The model under review builds one solid part; all positions refer to its coordinate system, in mm. Face numbers are marked on the shaded views. Round coordinates to 2 decimals unless told otherwise and drop trailing zeros. Order: outer loops, then holes, each group sorted by start corner. A loop starts at its lowest first (then second) coordinate and runs counter-clockwise, first axis right, second up. Notation, with made-up numbers: M 2.25,42.25 L 61.25,42.25 A23 cw 61.25,55.25 Z; hole C -25,-8.5 d7. An arc over 180 degrees is marked long. One line per item, written item: value. Start each with the question number.
from build123d import *

# Parameters (mm, degrees)
F0_R     = 1.6
F1_DEPTH = 3.175


with BuildPart() as f1:
    # F0 (on Top) → F1 (new body)
    with BuildSketch(Plane.XY):
        with BuildLine():
            Line((38.1, 6.35), (0, 6.35))
            ThreePointArc((0, 6.35), (-4.490128, 4.490128), (-6.35, 0))
            ThreePointArc((-6.35, 0), (-4.490128, -4.490128), (0, -6.35))
            Line((0, -6.35), (38.1, -6.35))
            ThreePointArc((38.1, -6.35), (42.590128, -4.490128), (44.45, 0))
            ThreePointArc((44.45, 0), (42.590128, 4.490128), (38.1, 6.35))
        make_face()
        with Locations((8.1, -3.175)):
            Circle(F0_R, mode=Mode.SUBTRACT)
        with Locations((18.1, -3.175)):
            Circle(F0_R, mode=Mode.SUBTRACT)
        with Locations((28.1, -3.175)):
            Circle(F0_R, mode=Mode.SUBTRACT)
        with Locations((38.1, -3.175)):
            Circle(F0_R, mode=Mode.SUBTRACT)
        Polygon((-2.313127, 1.150841), (-2.481189, 1.651718), (-1.954254, 1.689937), (-1.992473, 2.216873), (-1.472587, 2.122848), (-1.378562, 2.642733), (-0.898392, 2.422372), (-0.678031, 2.902541), (-0.267748, 2.56969), (0.065104, 2.979972), (0.37972, 2.555544), (0.804147, 2.87016), (1.003328, 2.380825), (1.492663, 2.580005), (1.563894, 2.056509), (2.08739, 2.12774), (2.026194, 1.602976), (2.550958, 1.54178), (2.361181, 1.048721), (2.85424, 0.858945), (2.547807, 0.428572), (2.97818, 0.122139), (2.574344, -0.218506), (2.914989, -0.622342), (2.439126, -0.851855), (2.668639, -1.327718), (2.150649, -1.431678), (2.254609, -1.949669), (1.727038, -1.921544), (1.698914, -2.449115), (1.194912, -2.290672), (1.036469, -2.794674), (0.587704, -2.515869), (0.308899, -2.964634), (-0.056431, -2.582985), (-0.43808, -2.948314), (-0.69702, -2.487802), (-1.157533, -2.746742), (-1.293813, -2.236301), (-1.804254, -2.372581), (-1.809311, -1.844285), (-2.337607, -1.849342), (-2.211123, -1.336386), (-2.724079, -1.209903), (-2.474002, -0.744517), (-2.939388, -0.494441), (-2.581431, -0.105868), (-2.970004, 0.252089), (-2.526659, 0.539434), (-2.814004, 0.982779), align=None, mode=Mode.SUBTRACT)
        with Locations((8.1, 3.175)):
            Circle(F0_R, mode=Mode.SUBTRACT)
        with Locations((18.1, 3.175)):
            Circle(F0_R, mode=Mode.SUBTRACT)
        with Locations((28.1, 3.175)):
            Circle(F0_R, mode=Mode.SUBTRACT)
        with Locations((38.1, 3.175)):
            Circle(F0_R, mode=Mode.SUBTRACT)
    extrude(amount=F1_DEPTH)


solid = f1.part
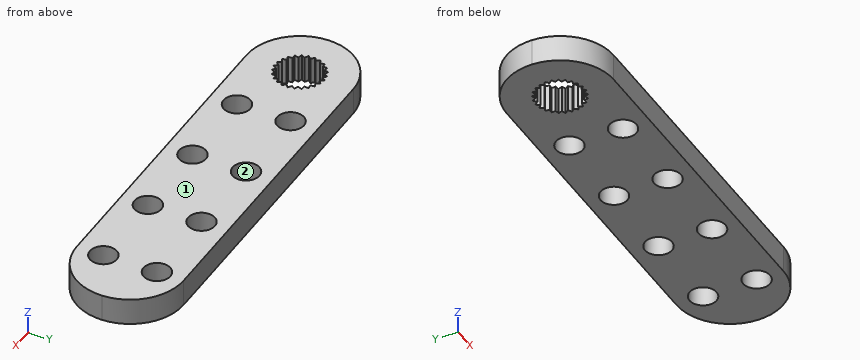
Item 1: Consider section A-A, the plane x = 18.1. Give the boundary of the cut face in (y, z) (3 decimals), then the cut area to 3 significant figures.
Item 2: Consider section B-B, the plane y = -4. Give the boundary of the cut face in (x, z) (3 decimals).
Item 3: Consider section C-C, the plane z = 0.85. Count the separate pieces of the cut face and the enclosed holes in it, then the cut area to 3 significant figures.
Item 4: Clearance check with flat-ended pins moving along their axes: P1, Ø1.9, axis at x = 38.1, y = -3.175, coming from the +Z side; P2, Ø1.5, axis at y = 5, z = 0.5, coming from the -X side. State where each tip first meets the part, or that it passes through.
Item 5: Wall thickness on L1, parallel to Y at x = 38.1, z = 2.25 (3 decimals); L2, parallel to X at y = -4.25, z = 2.1: over which ranges is each line inside the solid? List them lowest first.
Item 6: The part is to be moulded in two halves that separate along X. For the marked faces 1 and 2, say which applies: pulls with the +X half, pulls with the -X half, needs draft (parallel to the pull), parting line crosses it, or undercut.
Computed:
1. outline: M -6.35,0 L -4.775,0 L -4.775,3.175 L -6.35,3.175 Z; M -1.575,0 L 1.575,0 L 1.575,3.175 L -1.575,3.175 Z; M 4.775,0 L 6.35,0 L 6.35,3.175 L 4.775,3.175 Z
1. area: 20.0 mm^2
2. outline: M -4.932,0 L 6.729,0 L 6.729,3.175 L -4.932,3.175 Z; M 9.471,0 L 16.729,0 L 16.729,3.175 L 9.471,3.175 Z; M 19.471,0 L 26.729,0 L 26.729,3.175 L 19.471,3.175 Z; M 29.471,0 L 36.729,0 L 36.729,3.175 L 29.471,3.175 Z; M 39.471,0 L 43.032,0 L 43.032,3.175 L 39.471,3.175 Z
3. separate pieces: 1
3. enclosed holes: 9
3. area: 522 mm^2
4. P1: passes through
4. P2: stops at x = -4.72
5. L1: y = -6.35 to -4.775, -1.575 to 1.575, 4.775 to 6.35
5. L2: x = -4.72 to 6.91, 9.29 to 16.91, 19.29 to 26.91, 29.29 to 36.91, 39.29 to 42.82
6. face 1: needs draft
6. face 2: undercut
